The model under review builds one solid part; all positions refer to its coordinate system, in mm. Face numbers are marked on the shaded views. A direction names the side the tool comes from. Round coordinates to 2 decimals unless told otherwise and drop trailing zeros. Loops run counter-clockwise (first coordinate to the right, second up) from the corner with the lowest first, then second, coordinate; pieces in that order, holes last. Notation, with made-up numbers: (9.5, 68) -> (65.5, 68) arc R22 ccw to (65.5, 92) -> close; hole circle Ø9 at (-7.75, 54). An arc over 180 degrees is marked (long way). Use a Markdown table: item, result. Add a question column.
1) Insertion check: pin 1 (10.5 mm diameter, centred on y = 1, z = 14, fed in from +X); pin 2 (6 mm diameter, centred on y = 0, z = 12.5, fed in from +X); pin 3 (9 mm diameter, centred on y = -35, z = 12.5, fed in from -X) (3 decimals). Each pin has a flat end and moves straight along its axis. Give the tip position at first contact, or say it passes through.
2) For the marked faces 4, 5, 6 and 7, list the 3-axis set-ups (+Z, -Z, +X, -X, +Y, -Y) from which the entire face can be reached by the end or side of a thin tool; tool diameter is ignored.
3) Consider section D-D on x = -12. Give the boundary of the cut face in (y, z), plus the area to 3 significant figures.
4) Mouldability with a two-part tool opening along Y and no side actions: class the marked faces 1, 2 and 3 as released by +Y, released by -Y, zero draft, split by the parting line, or undercut.
5) Consider section A-A on x = 1. Give the boundary of the cut face in (y, z), plus the area to 3 significant figures.
6) Wall thickness on probe 1 along Y at (x, z) = (-4, 12.5); probe 2 along Y at (x, z) = (3, 7); probe 3 along Z at (x, y) = (-27, -35): over which ranges is each line inside the solid? List them lowest first.
7) Consider section B-B on y = -35. Give the boundary of the cut face in (x, z) (3 decimals).
8) Consider section C-C on z = 12.5. State how many separate pieces and enclosed holes the cut face has, plus the area to 3 significant figures.
from build123d import *

# Parameters (mm, degrees)
BOSS_EXTRUDE1_DEPTH                              = 25
SKETCH3_R                                        = 4.8
CUT_EXTRUDE1_DEPTH                               = 7.5
FILLET1_R                                        = 5
CBORE_FOR_1_4_SOCKET_HEAD_CAP_SCREW1_D           = 6.5278
CBORE_FOR_1_4_SOCKET_HEAD_CAP_SCREW1_CBORE_D     = 11.1125
CBORE_FOR_1_4_SOCKET_HEAD_CAP_SCREW1_CBORE_DEPTH = 22.225


with BuildPart() as part:
    # Sketch2 → Boss-Extrude1 (new body)
    with BuildSketch(Plane.XY):
        Polygon((-18, 25), (18, 25), (18, 45), (-33, 45), (-33, -45), (18, -45), (18, -25), (-18, -25), align=None)
    extrude(amount=BOSS_EXTRUDE1_DEPTH)

    # Sketch3 → Cut-Extrude1 (cut)
    with BuildSketch(Plane(origin=(-18, 0, 0), x_dir=(0, 0, -1), z_dir=(1, 0, 0))):
        with Locations(Location((-12.5, 0, 0), (0, 0, 90))):
            Circle(SKETCH3_R)
    extrude(amount=-CUT_EXTRUDE1_DEPTH, mode=Mode.SUBTRACT)

    # Fillet1
    fillet1_edges = [part.edges().sort_by_distance(p)[0] for p in [
        (-33, -45, 12.5),
        (-33, 45, 12.5),
        (-18, 25, 12.5),
        (-18, -25, 12.5),
    ]]
    fillet(fillet1_edges, radius=FILLET1_R)

    # CBORE for 1/4 Socket Head Cap Screw1 (through all)
    with Locations(Plane.ZY.offset(33)):
        with Locations((12.5, 35), (12.5, -35)):
            CounterBoreHole(CBORE_FOR_1_4_SOCKET_HEAD_CAP_SCREW1_D / 2, CBORE_FOR_1_4_SOCKET_HEAD_CAP_SCREW1_CBORE_D / 2, CBORE_FOR_1_4_SOCKET_HEAD_CAP_SCREW1_CBORE_DEPTH)


solid = part.part
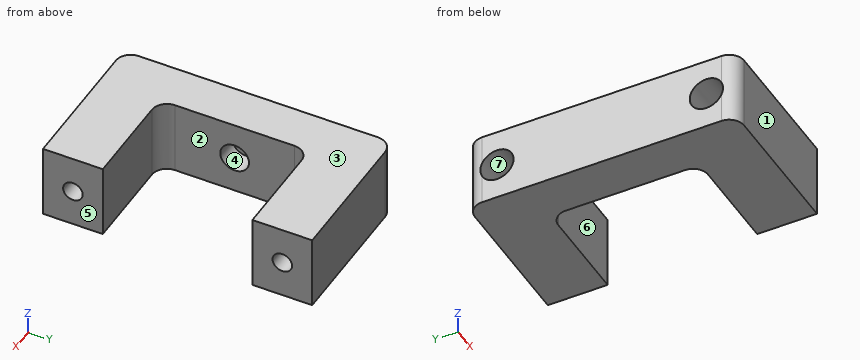
Result set:
| question | item | result |
|---|---|---|
| 1 | pin 1 | x = -18 |
| 1 | pin 2 | x = -25.5 |
| 1 | pin 3 | x = -10.775 |
| 2 | face 4 | +X |
| 2 | face 5 | +Z, -Z, +X, +Y, -Y |
| 2 | face 6 | +Z, -Z, +X |
| 2 | face 7 | -X |
| 3 | outline | (-45, 0) -> (-25, 0) -> (-25, 25) -> (-45, 25) -> close; (25, 0) -> (45, 0) -> (45, 25) -> (25, 25) -> close; hole circle Ø11.11 at (-35, 12.5); hole circle Ø11.11 at (35, 12.5) |
| 3 | area | 806 mm2 |
| 4 | face 1 | released by -Y |
| 4 | face 2 | undercut |
| 4 | face 3 | zero draft |
| 5 | outline | (-45, 0) -> (-25, 0) -> (-25, 25) -> (-45, 25) -> close; (25, 0) -> (45, 0) -> (45, 25) -> (25, 25) -> close; hole circle Ø6.53 at (-35, 12.5); hole circle Ø6.53 at (35, 12.5) |
| 5 | area | 933 mm2 |
| 6 | probe 1 | -45 to -38.26, -31.74 to -25, 25 to 31.74, 38.26 to 45 |
| 6 | probe 2 | -45 to -25, 25 to 45 |
| 6 | probe 3 | 0 to 6.94, 18.06 to 25 |
| 7 | outline | (-33, 0) -> (18, 0) -> (18, 9.236) -> (-10.775, 9.236) -> (-10.775, 6.944) -> (-33, 6.944) -> close; (-33, 18.056) -> (-10.775, 18.056) -> (-10.775, 15.764) -> (18, 15.764) -> (18, 25) -> (-33, 25) -> close |
| 8 | separate pieces | 3 |
| 8 | enclosed holes | 0 |
| 8 | area | 1,850 mm2 |
